from build123d import *

# Parameters (mm, degrees)
SKETCH_8_W          = 25
SKETCH_8_H          = 25
SKETCH_8_W_2        = 4
SKETCH_8_H_2        = 21
SKETCH_8_W_3        = 2
EXTRUDE_7_DEPTH     = 25
SKETCH_9_W          = 25
SKETCH_9_H          = 25
EXTRUDE_8_DEPTH     = 2
SKETCH_11_W         = 25
SKETCH_11_H         = 35
EXTRUDE_9_DEPTH     = 6
SKETCH_12_W         = 21
SKETCH_12_H         = 30
CUT_EXTRUDE_1_DEPTH = 4
SKETCH_14_W         = 25
SKETCH_14_H         = 1.5
EXTRUDE_11_DEPTH    = 25
SKETCH_15_W         = 25
SKETCH_15_H         = 35
EXTRUDE_12_DEPTH    = 2


with BuildPart() as part:
    # 草图8 → 凸台-拉伸7 (new body)
    with BuildSketch(Plane.XY):
        Rectangle(SKETCH_8_W, SKETCH_8_H)
        with Locations((3.5, 0)):
            Rectangle(SKETCH_8_W_2, SKETCH_8_H_2, mode=Mode.SUBTRACT)
        with Locations((-3.5, 0)):
            Rectangle(SKETCH_8_W_2, SKETCH_8_H_2, mode=Mode.SUBTRACT)
        with Locations((-9.5, 0)):
            Rectangle(SKETCH_8_W_3, SKETCH_8_H_2, mode=Mode.SUBTRACT)
        with Locations((9.5, 0)):
            Rectangle(SKETCH_8_W_3, SKETCH_8_H_2, mode=Mode.SUBTRACT)
    extrude(amount=EXTRUDE_7_DEPTH)

    # 草图9 → 凸台-拉伸8 (add)
    with BuildSketch(Plane(origin=(0, 0, 0), x_dir=(-1, 0, 0), z_dir=(0, 0, -1))):
        Rectangle(SKETCH_9_W, SKETCH_9_H)
    extrude(amount=EXTRUDE_8_DEPTH)

    # 草图11 → 凸台-拉伸9 (add)
    with BuildSketch(Plane(origin=(0, 0, -2), x_dir=(-1, 0, 0), z_dir=(0, 0, -1))):
        Rectangle(SKETCH_11_W, SKETCH_11_H)
    extrude(amount=EXTRUDE_9_DEPTH)

    # 草图12 → 切除-拉伸1 (cut)
    with BuildSketch(Plane(origin=(0, 0, -8), x_dir=(-1, 0, 0), z_dir=(0, 0, -1))):
        Rectangle(SKETCH_12_W, SKETCH_12_H)
    extrude(amount=-CUT_EXTRUDE_1_DEPTH, mode=Mode.SUBTRACT)

    # 草图14 → 凸台-拉伸11 (add)
    with BuildSketch(Plane.XY.offset(25)):
        Rectangle(SKETCH_14_W, SKETCH_14_H)
        with Locations((0, 6)):
            Rectangle(SKETCH_14_W, SKETCH_14_H)
        with Locations((0, -6)):
            Rectangle(SKETCH_14_W, SKETCH_14_H)
    extrude(amount=-EXTRUDE_11_DEPTH)

    # 草图15 → 凸台-拉伸12 (add)
    with BuildSketch(Plane(origin=(0, 0, -8), x_dir=(-1, 0, 0), z_dir=(0, 0, -1))):
        Rectangle(SKETCH_15_W, SKETCH_15_H)
    extrude(amount=EXTRUDE_12_DEPTH)


solid = part.part
Build history of the part. All positions in model axes, mm. A direction names the side the tool comes from. Give positions to 0.01 mm unless a question says otherwise; leave off trailing zeros. Write each loop counter-clockwise with the first axis right and the second up, starting at its lowest first coordinate (ties: lowest second). Pieces come first, ordered by that corner, then holes. Notation, with made-up numbers: (-38, 23.5) - (2, 23.5) arc R26 cw to (2, 50.5) - close; hole circle Ø5 at (40.25, 58.5). An arc over 180 degrees is marked (long way). Use one line per item in the form item = value. Start each with the question number.
1. Band-saw the part on D-D on x = 11. Write the cut outline in (y, z), plus the area to 3 significant figures.
2. Band-saw the part on B-B on y = -13. Write the cut outline in (x, z), plus the area to 3 significant figures.
3. 3-axis set-ups, long thin cutter, end or side, ignore diameter. For faces 1 (the face through (-10, 5.25, 13)), 2 (the face through (0, -17.5, -6)), 3 (the face through (-10.5, 0, -6)): which of +Z, -Z, +X, -X, +Y, -Y reach the whole face in a straight line?
4. Band-saw the part on C-C on x = -6. Write the cut outline in (y, z).
5. Band-saw the part on A-A on z = -6. Write the cut outline in (x, y).
6. Probe line 1 (X direction, y = -7.5, z = 22.5); line 2 (Y direction, x = -5.25, z = 17); line 3 (Z direction, x = -5.25, y = -11.5). List the from-to ranges inside material, lowest first. Write a range as [from, to].
7. Two-plate mould, pull along X, no slides. Class faces 4 (the face through (-10, 6.75, 13)), 5 (the face through (0, 17.5, -6)): released by +X, released by -X, zero draft, split by the parting line, or undercut.
8. Drop flat-ended pins along their axis: pin 1 Ø1.2 at (x, y) = (2.5, 2) entering from +Z; pin 2 Ø4.5 at (x, z) = (3, 10.5) entering from -Y; pin 3 Ø0.6 at (x, z) = (-10, 13) entering from +Y. Give the stop position or say it passes through.
Conclusion:
q1.outline = (-17.5, -10) - (17.5, -10) - (17.5, -2) - (12.5, -2) - (12.5, 25) - (-12.5, 25) - (-12.5, -2) - (-17.5, -2) - close
q1.area = 955 mm²
q2.outline = (-12.5, -10) - (12.5, -10) - (12.5, -2) - (-12.5, -2) - close; hole (-10.5, -8) - (10.5, -8) - (10.5, -4) - (-10.5, -4) - close
q2.area = 116 mm²
q3.face_1 = +Z
q3.face_2 = +Z, -Z, +X, -X, -Y
q3.face_3 = none
q4.outline = (-17.5, -10) - (17.5, -10) - (17.5, -2) - (12.5, -2) - (12.5, 25) - (-12.5, 25) - (-12.5, -2) - (-17.5, -2) - close; hole (-15, -8) - (15, -8) - (15, -4) - (-15, -4) - close
q5.outline = (-12.5, -17.5) - (12.5, -17.5) - (12.5, 17.5) - (-12.5, 17.5) - close; hole (-10.5, -15) - (10.5, -15) - (10.5, 15) - (-10.5, 15) - close
q6.line_1 = [-12.5, -10.5], [-8.5, -5.5], [-1.5, 1.5], [5.5, 8.5], [10.5, 12.5]
q6.line_2 = [-12.5, -10.5], [-6.75, -5.25], [-0.75, 0.75], [5.25, 6.75], [10.5, 12.5]
q6.line_3 = [-10, -8], [-4, 25]
q7.face_4 = undercut
q7.face_5 = zero draft
q8.pin_1 = 0
q8.pin_2 = -12.5
q8.pin_3 = 12.5
